Autodesk Inventor part; units mm, degrees
ref_plane "YZ Plane" through (0, 0, 0) normal (1, 0, 0) x (0, 1, 0)
ref_plane "XY Plane" through (0, 0, 0) normal (0, 0, 1) x (1, 0, 0)
sketch "スケッチ2" plane through (0, 0, 0) normal (0, 0, 1) x (1, 0, 0)
  line L0 (2279, 0) -> (2279, 1939)
  line L1 (0, 1939.0001) -> (183.5291, 1939.0001)
  line L2 (183.5291, 1939.0001) -> (183.5291, 183.5291)
  line L3 (183.5291, 0) -> (0, 0)
  line L4 (0, 0) -> (0, 1939.0001)
  line L5 (0, 0) -> (2279, 0)
  line L6 (2279, 0) -> (2279, 183.5291)
  line L7 (2095.4709, 183.5291) -> (183.5291, 183.5291)
  line L8 (0, 183.5291) -> (0, 0)
  line L9 (2279, 0) -> (2095.4709, 0)
  line L10 (2095.4709, 183.5291) -> (2095.4709, 1939)
  line L11 (2095.4709, 1939) -> (2279, 1939)
  line L12 (2279, 1939) -> (2279, 0)
  line L13 (2279, 1939) -> (2095.4709, 1939)
  line L14 (183.5291, 1939.0001) -> (0, 1939.0001)
  dimension "d10" = 2279
  dimension "d11" = 1939
  dimension "d12" = 1755.4709
  dimension "d13" = 1755.471
extrude "押し出し1" add sketch "スケッチ2" along normal blind 170
properties part number "rail"
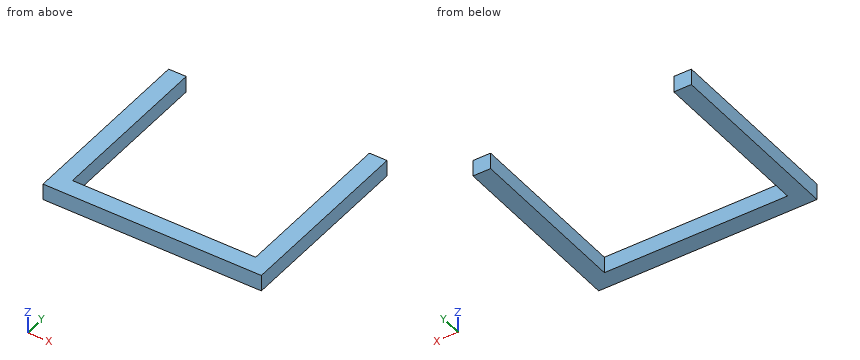
Check sheet for the modelled part. Datum: model origin and axes. Units: mm. Give positions to 0.01 mm unless a question says otherwise; leave off trailing zeros. Loops run counter-clockwise (first coordinate to the right, second up) from the corner with the lowest first, then second, coordinate; pieces in that order, holes last. Notation, with made-up numbers: M 52.25,83.5 L 62.25,83.5 A22 ccw 62.25,104.5 Z; hole C 58,-4 d10. An arc over 180 degrees is marked long. Use a Markdown table: item, result. Add a question column.
Q1. Go/stop test with flat-tipped pins: pin 1 (3 mm diameter, centred on y = 1143.5, z = 73, fed in from -X); pin 2 (1.5 mm diameter, centred on x = 322, z = 28, fed in from +Y). Record where each tip stops, or that it passes through.
Q2. Scan lines: line 1 along X through (y, z) = (1585, 131); line 2 along Y through (x, z) = (280.5, 104). Record each from-to range of solid material in increasing order. Write a range as [from, to].
Q3. Sectioned sample at C-C, the plane x = 457. Record the cut outline in (y, z).
Q4. Sectioned sample at B-B, the plane z = 44.5. Record the cut outline in (x, y), then the cut area to 3 significant figures.
Q5. Sectioned sample at A-A, the plane y = 1672. Record the cut outline in (x, z), then the cut area to 3 significant figures.
Verdict:
| question | item | result |
|---|---|---|
| 1 | pin 1 | x = 0 |
| 1 | pin 2 | y = 183.53 |
| 2 | line 1 | [0, 183.53], [2095.47, 2279] |
| 2 | line 2 | [0, 183.53] |
| 3 | outline | M 0,0 L 183.53,0 L 183.53,170 L 0,170 Z |
| 4 | outline | M 0,0 L 2279,0 L 2279,1939 L 2095.47,1939 L 2095.47,183.53 L 183.53,183.53 L 183.53,1939 L 0,1939 Z |
| 4 | area | 1,060,000 mm^2 |
| 5 | outline | M 0,0 L 183.53,0 L 183.53,170 L 0,170 Z; M 2095.47,0 L 2279,0 L 2279,170 L 2095.47,170 Z |
| 5 | area | 62,400 mm^2 |
